Solid Edge part; units mm, degrees
sketch "Sketch1" plane through (0, 0, 0) normal (0, 0, 1) x (1, 0, 0)
  arc A0 (-1.6, 0) -> (-0.9285, 1.9613) centre (1.6, 0) cw
  arc A1 (-0.9285, 1.9613) -> (-0.8495, 2) centre (-0.8495, 1.9) cw
  line L0 (-0.8495, 2) -> (0, 2)
  line L1 (0, 2) -> (0, 1.2)
  arc A2 (0, 1.2) -> (0.1, 1.1) centre (0.1, 1.2) ccw
  line L2 (0.1, 1.1) -> (2.5, 1.1)
  line L3 (2.5, 1.1) -> (4.5, 0)
  line L4 (4.5, 0) -> (-1.6, 0)
revolve "RevolvedProtrusion1" add sketch "Sketch1" angle 360 about axis through (4.5, 0, 0) along (-1, 0, 0)
cosmetic_thread "Thread1"
sketch "Sketch2" plane through (-1.6, 0, 0) normal (1, 0, 0) x (0, 1, 0)
  line L0 (0.2375, 0.95) -> (-0.2375, 0.95)
  line L1 (-0.2375, 0.95) -> (-0.1876, 0.38)
  line L2 (-0.1876, 0.38) -> (-0.2375, 0.2375)
  line L3 (-0.2375, 0.2375) -> (-0.38, 0.1876)
  line L4 (-0.38, 0.1876) -> (-0.95, 0.2375)
  line L5 (-0.95, 0.2375) -> (-0.95, -0.2375)
  line L6 (-0.95, -0.2375) -> (-0.38, -0.1876)
  line L7 (-0.38, -0.1876) -> (-0.2375, -0.2375)
  line L8 (-0.2375, -0.2375) -> (-0.1876, -0.38)
  line L9 (-0.1876, -0.38) -> (-0.2375, -0.95)
  line L10 (-0.2375, -0.95) -> (0.2375, -0.95)
  line L11 (0.2375, -0.95) -> (0.1876, -0.38)
  line L12 (0.1876, -0.38) -> (0.2375, -0.2375)
  line L13 (0.2375, -0.2375) -> (0.38, -0.1876)
  line L14 (0.38, -0.1876) -> (0.95, -0.2375)
  line L15 (0.95, -0.2375) -> (0.95, 0.2375)
  line L16 (0.95, 0.2375) -> (0.38, 0.1876)
  line L17 (0.38, 0.1876) -> (0.2375, 0.2375)
  line L18 (0.2375, 0.2375) -> (0.1876, 0.38)
  line L19 (0.1876, 0.38) -> (0.2375, 0.95)
extrude "ExtrudedCutout_1" cut sketch "Sketch2" along normal blind 0.8
properties part number "SFS FN 362 310412 Blechschraube ISO 7049 Stahl einsatzgehärtet   verzinkt blau ST2.2x4.5-C-H"
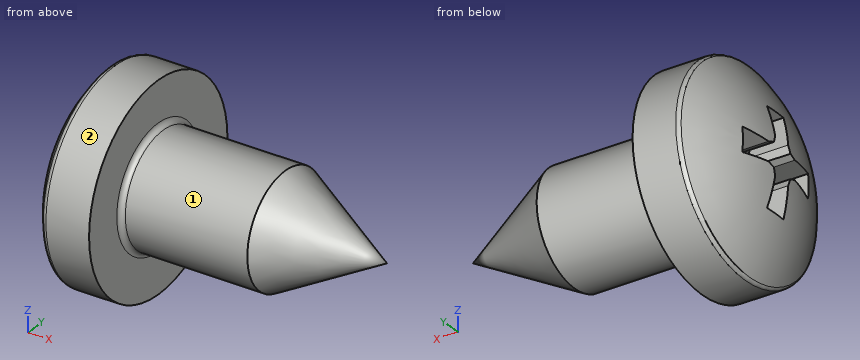
Read the model definition and answer for the solid it produces. Units are mm, in the model's axes. Face numbers are marked on the shaded views. A direction names the side the tool comes from. Coordinates: 2 decimals unless noted, no trailing zeros. Write each loop counter-clockwise with the first axis right and the second up, starting at its lowest first coordinate (ties: lowest second). Pieces come first, ordered by that corner, then holes. Notation, with made-up numbers: (18, 23.5) - (40, 23.5) arc R13 ccw to (40, 35.5) - close; hole circle Ø4 at (49.5, 67.5). An arc over 180 degrees is marked (long way). Answer as a JSON object with one key per item and string values. Group by question number.
1. Which of the six approach directions +Z, -Z, +X, -X, +Y, -Y give full straight-line access (tool end or side, diameter ignored) to the marked faces 1 and 2?
2. Consider L1, parallel to X at y = -1.2, z = -1.25; L2, parallel to Z at x = -0.75, y = 1.45; L3, parallel to X at y = 1.05, z = -1.65. Determine where each line is inside the solid, lowest interval first. Write a range as [from, to].
3. Each of these flat-tipped pins is pushed along its axis until it touches: P1, Ø2, axis at y = 1, z = -1, coming from the +X side; P2, Ø1.5, axis at x = 1.5, z = -0.5, coming from the +Y side; P3, Ø1.5, axis at x = 0, z = 1, coming from the -Y side. Where does it stop, or does it pass through?
4. A cutting plane is placed at A-A (x = 0.25). Determine the outline of the cut face in (y, z), plus the area to 3 significant figures.
Worked out:
{
 "1": {"face 1": "+X", "face 2": "+X, -X"},
 "2": {"L1": "x = [-1.09, 0]", "L2": "z = [-1.38, 1.38]", "L3": "x = [-0.93, 0]"},
 "3": {"P1": "stops at x = 3.75", "P2": "stops at y = 1.1", "P3": "stops at y = -1.98"},
 "4": {"outline": "circle Ø2.2 at (0, 0)", "area": "3.80 mm²"}
}
